Geometry check sheet. Reference: the model listing, model coordinates, mm. Face numbers are marked on the shaded views. A direction names the side the tool comes from. Round coordinates to 2 decimals unless told otherwise and drop trailing zeros. Loops run counter-clockwise (first coordinate to the right, second up) from the corner with the lowest first, then second, coordinate; pieces in that order, holes last. Notation, with made-up numbers: M 46,41.25 L 80,41.25 A28 ccw 80,77.25 Z; hole C 7,83.5 d9. An arc over 180 degrees is marked long. Use one line per item in the form item = value. Start each with the question number.
1. Material ranges on line 1 (Z direction, x = -5.5, y = 15); line 2 (Z direction, x = -11, y = -11.5), recorded low to high.
2. Set-up check for the marked faces 1 and 2: record each of +Z, -Z, +X, -X, +Y, -Y from which the full face is reachable in a straight line by a thin tool's end or side.
3. Go/stop test with flat-tipped pins: pin 1 (0.6 mm diameter, centred on x = -5.5, y = -9.5, fed in from +Z); pin 2 (8 mm diameter, centred on y = -4, z = 7.5, fed in from +X); pin 3 (2 mm diameter, centred on x = 1.5, y = -0.5, fed in from +Z). Record where each tip stops, or that it passes through.
4. Cross-section at A-A (z = 9.75). State how many separate pieces and enclosed holes the cut face has, then the cut area to 3 significant figures.
5. Cross-section at B-B (x = 17.5). Record the boundary of the cut face in (y, z).
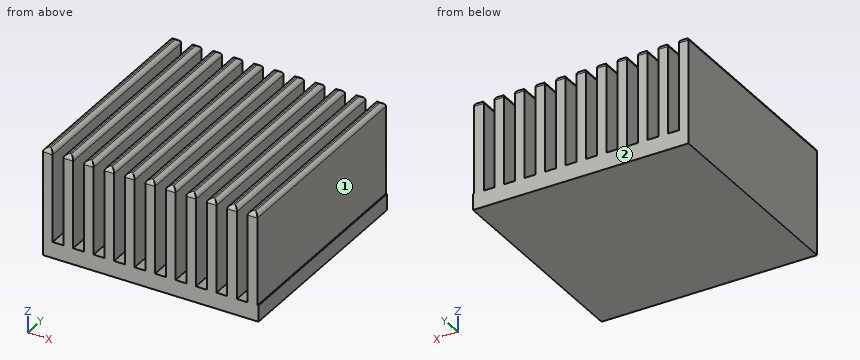
```python
from build123d import *

# Parameters (mm, degrees)
SKETCH1_W           = 40
SKETCH1_H           = 40
BOSS_EXTRUDE1_DEPTH = 3
SKETCH2_W           = 1.8
SKETCH2_H           = 40
BOSS_EXTRUDE2_DEPTH = 17
LPATTERN1_COUNT     = 11
LPATTERN1_PITCH     = 3.8
FILLET1_R           = 0.75


with BuildPart() as part:
    # Sketch1 → Boss-Extrude1 (new body)
    with BuildSketch(Plane.XY):
        Rectangle(SKETCH1_W, SKETCH1_H)
    extrude(amount=BOSS_EXTRUDE1_DEPTH)

    # Sketch2 → Boss-Extrude2 (add)
    with BuildSketch(Plane.XY.offset(3)):
        with Locations((-19.1, 0)):
            Rectangle(SKETCH2_W, SKETCH2_H)
    boss_extrude2 = extrude(amount=BOSS_EXTRUDE2_DEPTH)

    # LPattern1: Boss-Extrude2 ×11
    with Locations(*[(i * LPATTERN1_PITCH, 0, 0) for i in range(1, LPATTERN1_COUNT)]):
        add(boss_extrude2)

    # Fillet1
    fillet1_edges = [part.edges().sort_by_distance(p)[0] for p in [
        (10.4, 0, 20),
        (11.3, -20, 20),
        (12.2, 0, 20),
        (11.3, 20, 20),
        (14.2, 0, 20),
        (15.1, -20, 20),
        (16, 0, 20),
        (15.1, 20, 20),
        (18, 0, 20),
        (18.9, -20, 20),
        (19.8, 0, 20),
        (18.9, 20, 20),
        (-20, 0, 20),
        (-19.1, -20, 20),
        (-18.2, 0, 20),
        (-19.1, 20, 20),
        (-16.2, 0, 20),
        (-15.3, -20, 20),
        (-14.4, 0, 20),
        (-15.3, 20, 20),
        (-12.4, 0, 20),
        (-11.5, -20, 20),
        (-10.6, 0, 20),
        (-11.5, 20, 20),
        (-8.6, 0, 20),
        (-7.7, -20, 20),
        (-6.8, 0, 20),
        (-7.7, 20, 20),
        (-4.8, 0, 20),
        (-3.9, -20, 20),
        (-3, 0, 20),
        (-3.9, 20, 20),
        (-1, 0, 20),
        (-0.1, -20, 20),
        (0.8, 0, 20),
        (-0.1, 20, 20),
        (2.8, 0, 20),
        (3.7, -20, 20),
        (4.6, 0, 20),
        (3.7, 20, 20),
        (6.6, 0, 20),
        (7.5, -20, 20),
        (8.4, 0, 20),
        (7.5, 20, 20),
    ]]
    fillet(fillet1_edges, radius=FILLET1_R)


solid = part.part
```
Reported:
q1.line_1 = 0 to 3
q1.line_2 = 0 to 19.91
q2.face_1 = +Z, +X, +Y, -Y
q2.face_2 = +Z, -Z, +X, -X, +Y
q3.pin_1 = 3
q3.pin_2 = 19.8
q3.pin_3 = 19.85
q4.separate_pieces = 11
q4.enclosed_holes = 0
q4.area = 792 mm²
q5.outline = M -20,0 L 20,0 L 20,3 L -20,3 Z
